Input: dimensioned drawing with shaded views. Units: mm. Origin: part minimum x, y, z. A direction names the side the tool comes from. Round coordinates to 2 decimals unless told otherwise and drop trailing zeros. Loops run counter-clockwise (first coordinate to the right, second up) from the corner with the lowest first, then second, coordinate; pieces in that order, holes last. Notation, with made-up numbers: M 21.5,46.25 L 37.5,46.25 A10 cw 37.5,61.25 Z; hole C 85.25,48 d7. An arc over 180 degrees is marked long. Return JSON: item names as keys, results as strings.
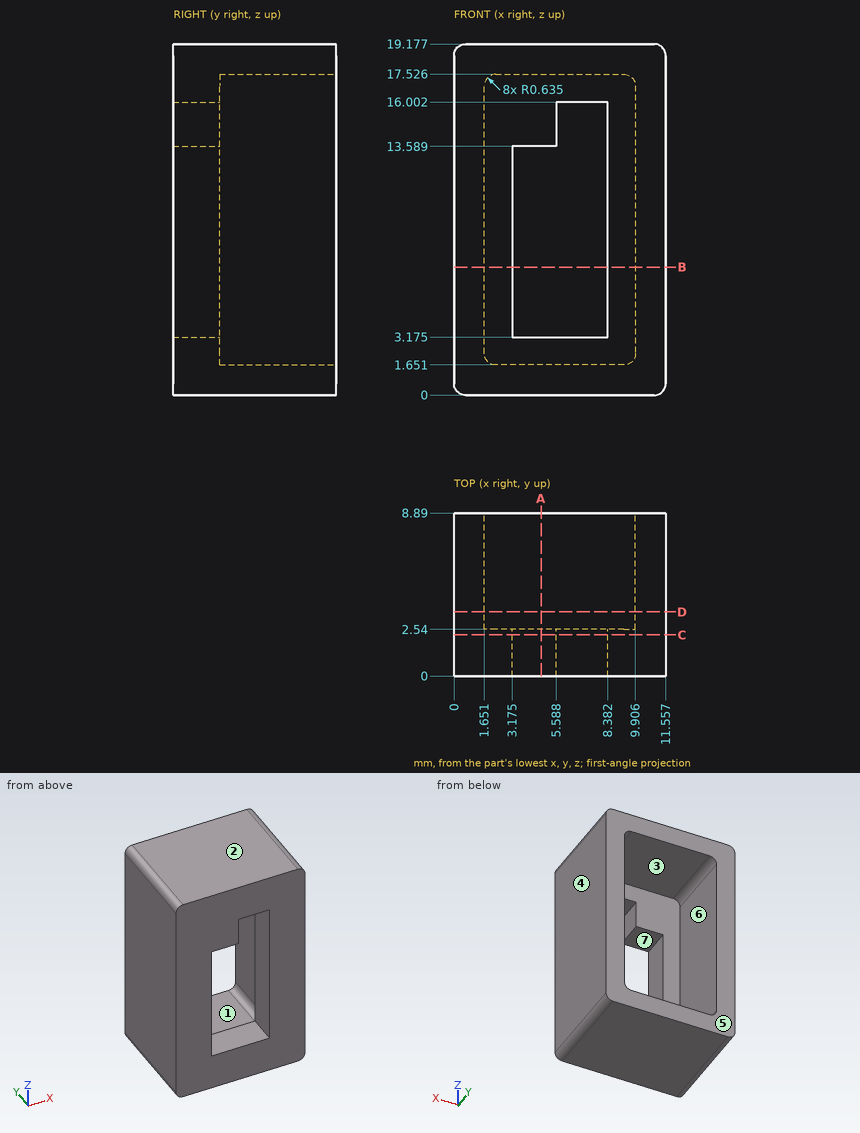
Q1. Pull-direction query (X, two-part tool) for the marked faces 1, 2, 3 and 4; classes: pulls with the +X half, pulls with the -X half, needs draft (parallel to the pull), parting line crosses it, or undercut.
Determined:
{"face 1": "undercut", "face 2": "needs draft", "face 3": "undercut", "face 4": "pulls with the +X half"}
Q2. Section query C-C (y = 2.25). Output: boundary loops of the cut face in (x, z) (3 decimals).
Determined:
{"outline": "M 0,0.635 A0.635 ccw 0.635,0 L 10.922,0 A0.635 ccw 11.557,0.635 L 11.557,18.542 A0.635 ccw 10.922,19.177 L 0.635,19.177 A0.635 ccw 0,18.542 Z; hole M 3.175,3.175 L 8.382,3.175 L 8.382,16.002 L 5.588,16.002 L 5.588,13.589 L 3.175,13.589 Z"}
Q3. Material intervals for L1, parallel to X at y = 8, z = 5; L2, parallel to X at y = 1, z = 4 (3 decimals); L3, parallel to Z at x = 2.25, y = 2.75, sorted ascending.
Determined:
{"L1": "x = 0 to 1.65, 9.91 to 11.56", "L2": "x = 0 to 3.175, 8.382 to 11.557", "L3": "z = 0 to 1.65, 17.52 to 19.18"}
Q4. Section query D-D (y = 3.5). Output: boundary loops of the cut face in (x, z) (3 decimals).
Determined:
{"outline": "M 0,0.635 A0.635 ccw 0.635,0 L 10.922,0 A0.635 ccw 11.557,0.635 L 11.557,18.542 A0.635 ccw 10.922,19.177 L 0.635,19.177 A0.635 ccw 0,18.542 Z; hole M 1.651,2.286 A0.635 ccw 2.286,1.651 L 9.271,1.651 A0.635 ccw 9.906,2.286 L 9.906,16.891 A0.635 ccw 9.271,17.526 L 2.286,17.526 A0.635 ccw 1.651,16.891 Z"}
Q5. Section query B-B (z = 7). Output: boundary loops of the cut face in (x, y) (3 decimals).
Determined:
{"outline": "M 0,0 L 3.175,0 L 3.175,2.54 L 1.651,2.54 L 1.651,8.89 L 0,8.89 Z; M 8.382,0 L 11.557,0 L 11.557,8.89 L 9.906,8.89 L 9.906,2.54 L 8.382,2.54 Z"}
Q6. Section query A-A (x = 4.75). Output: boundary loops of the cut face in (y, z) (3 decimals), plus the area to 3 significant figures.
Determined:
{"outline": "M 0,0 L 8.89,0 L 8.89,1.651 L 2.54,1.651 L 2.54,3.175 L 0,3.175 Z; M 0,13.589 L 2.54,13.589 L 2.54,17.526 L 8.89,17.526 L 8.89,19.177 L 0,19.177 Z", "area": "43.2 mm^2"}
Q7. Reachability of the marked faces 5, 6 and 7 from +Z, -Z, +X, -X, +Y, -Y: full face, straight path, thin tool, end or side. Return the list, or none.
Determined:
{"face 5": "+Z, -Z, +X, -X, +Y", "face 6": "+Y", "face 7": "+Y, -Y"}
